The listing builds one solid part. Answer for the finished solid, in the listing's coordinates (mm). Face numbers are marked on the shaded views. Coordinates: 2 decimals unless noted, no trailing zeros. Loops run counter-clockwise (first coordinate to the right, second up) from the corner with the lowest first, then second, coordinate; pieces in that order, holes last. Notation, with made-up numbers: M -15.5,-9 L 25.5,-9 A9 ccw 25.5,-4 Z; hole C -31.75,-25.5 d3. An arc over 180 degrees is marked long. Return JSON: item names as keys, results as strings. Group by question number.
1. Straight lines are drawn through the part: L1, parallel to Y at x = 0, z = 19.8; L2, parallel to Y at x = -0.25, z = 22. For each, find the intervals that lie inside material, in ascending order. Write a range as from..to.
2. The mould has two halves that part along X. Classify the marked faces 1, 2 and 3: pulls with the +X half, pulls with the -X half, needs draft (parallel to the pull), parting line crosses it, or undercut.
3. Section B-B (z = 28.5) is taken. Write down the section's boundary in (x, y), then the cut area to 3 significant figures.
4. Given P1, Ø9, axis at x = 0, y = 0, coming from the +Z side; P2, Ø2, axis at x = -1, y = -8, coming from the -Z side; P3, Ø5, axis at x = 5, y = 0.5, coming from the +Z side (3 decimals); P4, Ø1, axis at x = -6.5, z = 24, coming from the +Y side, each flat-ended and moving along its own axis, determine where each tip first touches the part or whether it passes through.
5. Section A-A (z = 17) is taken. Write down the section's boundary in (x, y).
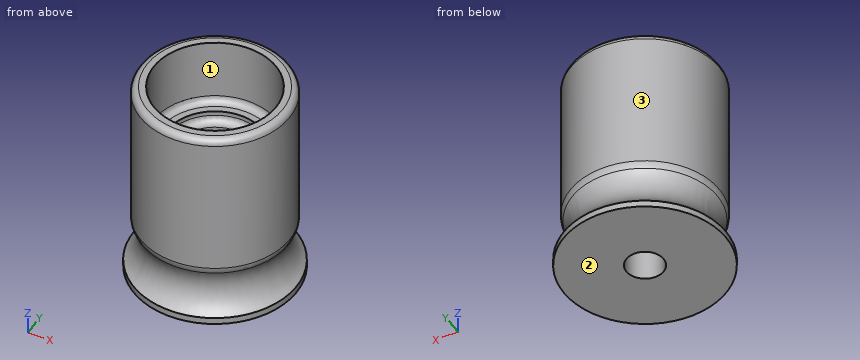
```python
from build123d import *

# Parameters (mm, degrees)
FILLET001_R  = 1
SKETCH010_R  = 2.75
POCKET_DEPTH = 30.326
FILLET002_R  = 2


with BuildPart() as part:
    # Sketch → Revolution (revolve)
    with BuildSketch(Plane.XZ):
        with BuildLine():
            Line((0, 0), (12, 0))
            Line((12, 0), (12, 1))
            ThreePointArc((11, 8), (10.050253, 4.292893), (12, 1))
            Line((11, 30.325), (11, 8))
            Line((9, 30.325), (11, 30.325))
            Line((9, 20.325), (9, 30.325))
            Line((7, 20.325), (9, 20.325))
            Line((7, 20.325), (7, 18.325))
            Line((0, 20.325), (7, 18.325))
            Line((0, 0), (0, 20.325))
        make_face()
    revolve(axis=Axis((0, 0, 0), (0, 0, 1)))

    # Fillet001
    fillet001_edges = [part.edges().sort_by_distance(p)[0] for p in [
        (-11, 0, 30.325),
        (-7, 0, 18.325),
        (-9, 0, 20.325),
    ]]
    fillet(fillet001_edges, radius=FILLET001_R)

    # Sketch010 (on Face4 of Fillet001) → Pocket (cut, through all)
    with BuildSketch(Plane(origin=(0, 0, 30.325), x_dir=(-1, 0, 0), z_dir=(0, 0, 1))):
        Circle(SKETCH010_R)
    extrude(amount=-POCKET_DEPTH, mode=Mode.SUBTRACT)

    # Fillet002
    fillet002_edges = [part.edges().sort_by_distance(p)[0] for p in [
        (-11, 0, 8),
    ]]
    fillet(fillet002_edges, radius=FILLET002_R)


solid = part.part
```
Worked out:
{
 "1": {"L1": "-11..-7, 7..11", "L2": "-11..-9, 9..11"},
 "2": {"face 1": "undercut", "face 2": "needs draft", "face 3": "parting line crosses it"},
 "3": {"outline": "C 0,0 d22; hole C 0,0 d18", "area": "126 mm^2"},
 "4": {"P1": "z = 19.54", "P2": "z = 0", "P3": "z = 20.325", "P4": "y = 9.22"},
 "5": {"outline": "C 0,0 d22; hole C 0,0 d5.5"}
}
